from build123d import *

# Parameters (mm, degrees)
F1_DEPTH = 1.27
F2_R     = 2.54
F3_DEPTH = 1.27
F4_R     = 1.27
F5_DEPTH = 0.762
F6_R     = 0.508


with BuildPart() as f1:
    # F0 (on Top) → F1 (new body)
    with BuildSketch(Plane.XY):
        with BuildLine():
            ThreePointArc((20.32, 14.732), (19.576051, 16.528051), (17.78, 17.272))
            Line((17.78, 17.272), (-17.78, 17.272))
            ThreePointArc((-17.78, 17.272), (-19.576051, 16.528051), (-20.32, 14.732))
            Line((-20.32, 14.732), (-20.32, -14.732))
            ThreePointArc((-20.32, -14.732), (-19.576051, -16.528051), (-17.78, -17.272))
            Line((-17.78, -17.272), (17.78, -17.272))
            ThreePointArc((17.78, -17.272), (19.576051, -16.528051), (20.32, -14.732))
            Line((20.32, -14.732), (20.32, 14.732))
        make_face()
    extrude(amount=F1_DEPTH)

    # F2 (on face) → F3 (join)
    with BuildSketch(Plane.XY.offset(1.27)):
        Circle(F2_R)
    extrude(amount=F3_DEPTH)

    # F4 (on face) → F5 (join)
    with BuildSketch(Plane.XY.offset(2.54)):
        Circle(F4_R)
    extrude(amount=F5_DEPTH)

    # F6
    f6_edges = [f1.edges().sort_by_distance(p)[0] for p in [
        (-2.54, 0, 2.54),
        (-1.27, 0, 3.302),
    ]]
    fillet(f6_edges, radius=F6_R)


solid = f1.part
Geometry check sheet. Reference: the model listing, model coordinates, mm. A direction names the side the tool comes from. Give positions to 0.01 mm unless a question says otherwise; leave off trailing zeros. Order: outer loops, then holes, each group sorted by start corner. A loop starts at its lowest first (then second) coordinate and runs counter-clockwise, first axis right, second up.
1. Access from +Z, -Z, +X, -X, +Y, -Y to the whole of each face (thin tool, end or side, straight path). Record for faces 1 (the face through (-0.33, 2.52, 1.65)), 2 (the face through (19.556, -16.548, 0.626)).
Completed:
face 1: +Z
face 2: +Z, -Z, +X, -Y
2. Sectioned sample at A-A (x = 0). Record the boundary of the cut face in (y, z), then the cut area to 3 significant figures.
Completed:
outline: (-17.27, 0) - (17.27, 0) - (17.27, 1.27) - (2.54, 1.27) - (2.54, 2.03) arc R0.51 ccw to (2.03, 2.54) - (1.27, 2.54) - (1.27, 2.79) arc R0.51 ccw to (0.76, 3.3) - (-0.76, 3.3) arc R0.51 ccw to (-1.27, 2.79) - (-1.27, 2.54) - (-2.03, 2.54) arc R0.51 ccw to (-2.54, 2.03) - (-2.54, 1.27) - (-17.27, 1.27) - close
area: 52.0 mm2
3. Depth check by flat-ended pin: pin 1 (8 mm diameter, centred on x = 6, y = -10.5, fed in from +Z). Enter the tip coordinate at first touch or a pass-through.
Completed:
pin 1: stops at z = 1.27
4. Sectioned sample at B-B (y = 10). Record the boundary of the cut face in (x, z), then the cut area to 3 significant figures.
Completed:
outline: (-20.32, 0) - (20.32, 0) - (20.32, 1.27) - (-20.32, 1.27) - close
area: 51.6 mm2
5. Scan lines: line 1 (X direction, y = 1, z = 2.9); line 2 (Z direction, x = -16, y = 13.5); line 3 (X direction, y = -16, z = 0.4). Record each from-to range of solid material in increasing order.
Completed:
line 1: x = -0.76 to 0.76
line 2: z = 0 to 1.27
line 3: x = -19.98 to 19.98
6. Sectioned sample at C-C (x = -7). Record the boundary of the cut face in (y, z), then the cut area to 3 significant figures.
Completed:
outline: (-17.27, 0) - (17.27, 0) - (17.27, 1.27) - (-17.27, 1.27) - close
area: 43.9 mm2
